Source: CAD feature listing. Evaluate the final solid. Frame: model axes, mm. Face numbers are marked on the shaded views. A direction names the side the tool comes from. Round coordinates to 2 decimals unless told otherwise and drop trailing zeros. Order: outer loops, then holes, each group sorted by start corner. A loop starts at its lowest first (then second) coordinate and runs counter-clockwise, first axis right, second up. Notation, with made-up numbers: (37.25, 53) - (59.25, 53) arc R21 cw to (59.25, 82) - close; hole circle Ø2 at (15, 10). An arc over 180 degrees is marked (long way). Put each result on its own line as item: value. Start each with the question number.
1) Section A-A on y = 68.5. Output: boundary loops of the cut face in (x, z) (3 decimals), then the cut area to 3 significant figures.
2) Section C-C on z = -45. Output: boundary loops of the cut face in (x, y) (3 decimals), then the cut area to 3 significant figures.
3) Section B-B on y = 31.75. Output: boundary loops of the cut face in (x, z) (3 decimals).
4) Contact query for flat-ended pins moving along their axis: P1, Ø14.5, axis at y = 26, z = -29.5, coming from the +X side (3 decimals); P2, Ø10, axis at x = 18.5, z = -8, coming from the -Y side; P3, Ø4, axis at x = 27.16, y = 6.35, coming from the +Z side; P4, Ø11.5, axis at x = 25, y = 41.5, coming from the -Z side (3 decimals). Output: stop coordinate, or through.
5) Access query for the marked faces 1 and 2. Directions: +Z, -Z, +X, -X, +Y, -Y. A direction counts if a zero-diameter tool reaches every point of the face in a straight line with its end or side. Return the directions, or none.
6) Line query: probe 1 along X at (y, z) = (73, -33) (3 decimals); probe 2 along Z at (x, y) = (5, 9.5) (3 decimals). Output: solid intervals per line, ascending. Write a range as [from, to].
7) Section D-D on x = 4.5. Output: boundary loops of the cut face in (y, z) (3 decimals).
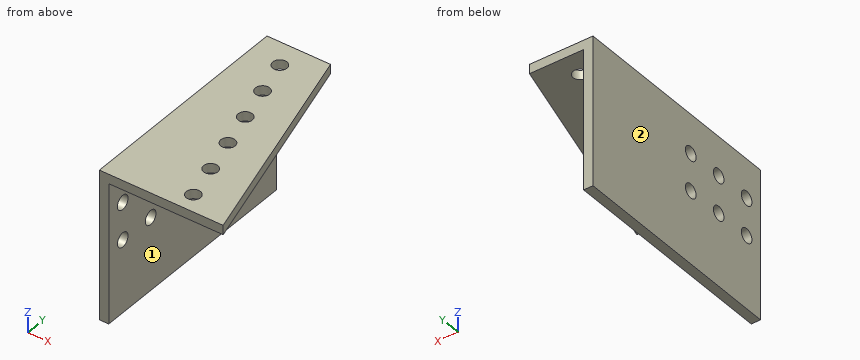
```python
from build123d import *

# Parameters (mm, degrees)
BOSS_EXTRUDE1_DEPTH = 76.2
SKETCH2_R           = 2.413
CUT_EXTRUDE1_DEPTH  = 104.224128115
SKETCH3_R           = 2.413
CUT_EXTRUDE2_DEPTH  = 100.4739202


with BuildPart() as part:
    # Sketch1 → Boss-Extrude1 (new body)
    with BuildSketch(Plane(origin=(0, 0, 0), x_dir=(1, 0, 0), z_dir=(0, 1, 0))):
        Polygon((0, 0), (0, 50.8), (3.175, 50.8), (3.175, 3.175), (50.8, 3.175), (50.8, 0), align=None)
    extrude(amount=BOSS_EXTRUDE1_DEPTH)

    # Sketch2 → Cut-Extrude1 (cut, through all)
    with BuildSketch(Plane(origin=(0, 0, -3.175), x_dir=(-1, 0, 0), z_dir=(0, 0, -1))):
        with Locations((-27.1582436, 6.35)):
            Circle(SKETCH2_R)
        with Locations((-23.871241727, 18.617257994)):
            Circle(SKETCH2_R)
        with Locations((-20.584239855, 30.884515988)):
            Circle(SKETCH2_R)
        with Locations((-17.297237982, 43.151773982)):
            Circle(SKETCH2_R)
        with Locations((-14.010236109, 55.419031975)):
            Circle(SKETCH2_R)
        with Locations((-10.723234236, 67.686289969)):
            Circle(SKETCH2_R)
        Polygon((-21.59, 76.2), (-50.8, -32.813204089), (-50.8, 76.2), align=None)
    extrude(amount=-CUT_EXTRUDE1_DEPTH, mode=Mode.SUBTRACT)

    # Sketch3 → Cut-Extrude2 (cut, through all)
    with BuildSketch(Plane(origin=(3.175, 0, 0), x_dir=(0, 0, -1), z_dir=(1, 0, 0))):
        with Locations((13.335, 6.35)):
            Circle(SKETCH3_R)
        with Locations((26.035, 6.35)):
            Circle(SKETCH3_R)
        with Locations((13.335, 19.05)):
            Circle(SKETCH3_R)
        with Locations((26.035, 19.05)):
            Circle(SKETCH3_R)
        with Locations((13.335, 31.75)):
            Circle(SKETCH3_R)
        with Locations((26.035, 31.75)):
            Circle(SKETCH3_R)
    extrude(amount=-CUT_EXTRUDE2_DEPTH, mode=Mode.SUBTRACT)


solid = part.part
```
Answer sheet:
1. outline: (0, -50.8) - (3.175, -50.8) - (3.175, -3.175) - (8.452, -3.175) - (8.452, 0) - (0, 0) - close; (12.995, -3.175) - (23.653, -3.175) - (23.653, 0) - (12.995, 0) - close
1. area: 212 mm^2
2. outline: (0, 0) - (3.175, 0) - (3.175, 76.2) - (0, 76.2) - close
2. area: 242 mm^2
3. outline: (0, -50.8) - (3.175, -50.8) - (3.175, -28.448) - (0, -28.448) - close; (0, -23.622) - (3.175, -23.622) - (3.175, -15.748) - (0, -15.748) - close; (0, -10.922) - (3.175, -10.922) - (3.175, -3.175) - (18.332, -3.175) - (18.332, 0) - (0, 0) - close; (22.837, -3.175) - (33.5, -3.175) - (33.5, 0) - (22.837, 0) - close
4. P1: x = 3.175
4. P2: y = 0
4. P3: through
4. P4: z = -3.175
5. face 1: -Z, +X, +Y, -Y
5. face 2: +Z, -Z, -X, +Y, -Y
6. probe 1: [0, 3.175]
6. probe 2: [-3.175, 0]
7. outline: (0, -3.175) - (76.2, -3.175) - (76.2, 0) - (0, 0) - close
